Source: CAD feature listing. Evaluate the final solid. Frame: model axes, mm. A direction names the side the tool comes from. Give positions to 0.01 mm unless a question says otherwise; leave off trailing zeros. Order: outer loops, then holes, each group sorted by start corner. A loop starts at its lowest first (then second) coordinate and runs counter-clockwise, first axis right, second up.
from build123d import *

# Parameters (mm, degrees)
PARED_Y_1_4IN_START          = -101.6
CROQUIS1_W                   = 228.6
CROQUIS1_H                   = 50.8
PARED_Y_1_4IN_DEPTH          = 6.35
ROSCA_M3_INFERIOR_START      = 12.7
CROQUIS2_R                   = 1.25
ROSCA_M3_INFERIOR_DEPTH      = 10
ROSCA_M3_SUPERIOR_START      = 53.5
CROQUIS3_R                   = 1.25
ROSCA_M3_SUPERIOR_DEPTH      = 10
BARRENOS_M3_ESQUINAS_START   = -101.6
CROQUIS4_R                   = 1.7
BARRENOS_M3_ESQUINAS_DEPTH   = 6.35
REFRENTADO_M3_ESQUINAS_START = -101.6
CROQUIS5_R                   = 2.9
REFRENTADO_M3_ESQUINAS_DEPTH = 3.2
VENTANA_PUERTOS_RPI5_START   = -101.6
VENTANA_PUERTOS_RPI5_DEPTH   = 6.35
RANURAS_VENTILACION_START    = -101.6
RANURAS_VENTILACION_DEPTH    = 6.35


with BuildPart() as part:
    # Croquis1 → Pared_-Y_1-4in (new body)
    with BuildSketch(Plane(origin=(0, 0, 0), x_dir=(1, 0, 0), z_dir=(0, 1, 0)).offset(PARED_Y_1_4IN_START)):
        with Locations((-25.4, -38.1)):
            Rectangle(CROQUIS1_W, CROQUIS1_H)
    extrude(amount=PARED_Y_1_4IN_DEPTH)

    # Croquis2 → Rosca_M3_inferior (cut)
    with BuildSketch(Plane.XY.offset(ROSCA_M3_INFERIOR_START)):
        with Locations((-125, -98.425)):
            Circle(CROQUIS2_R)
        with Locations((-30, -98.425)):
            Circle(CROQUIS2_R)
        with Locations((70, -98.425)):
            Circle(CROQUIS2_R)
    extrude(amount=ROSCA_M3_INFERIOR_DEPTH, mode=Mode.SUBTRACT)

    # Croquis3 → Rosca_M3_superior (cut)
    with BuildSketch(Plane.XY.offset(ROSCA_M3_SUPERIOR_START)):
        with Locations((-125, -98.425)):
            Circle(CROQUIS3_R)
        with Locations((-30, -98.425)):
            Circle(CROQUIS3_R)
        with Locations((70, -98.425)):
            Circle(CROQUIS3_R)
    extrude(amount=ROSCA_M3_SUPERIOR_DEPTH, mode=Mode.SUBTRACT)

    # Croquis4 → Barrenos_M3_esquinas (cut)
    with BuildSketch(Plane(origin=(0, 0, 0), x_dir=(1, 0, 0), z_dir=(0, 1, 0)).offset(BARRENOS_M3_ESQUINAS_START)):
        with Locations(Location((-136.525, -25, 0), (0, 0, 270))):
            Circle(CROQUIS4_R)
        with Locations(Location((-136.525, -50, 0), (0, 0, 270))):
            Circle(CROQUIS4_R)
        with Locations(Location((85.725, -25, 0), (0, 0, 270))):
            Circle(CROQUIS4_R)
        with Locations(Location((85.725, -50, 0), (0, 0, 270))):
            Circle(CROQUIS4_R)
    extrude(amount=BARRENOS_M3_ESQUINAS_DEPTH, mode=Mode.SUBTRACT)

    # Croquis5 → Refrentado_M3_esquinas (cut)
    with BuildSketch(Plane(origin=(0, 0, 0), x_dir=(1, 0, 0), z_dir=(0, 1, 0)).offset(REFRENTADO_M3_ESQUINAS_START)):
        with Locations(Location((-136.525, -25, 0), (0, 0, 270))):
            Circle(CROQUIS5_R)
        with Locations(Location((-136.525, -50, 0), (0, 0, 270))):
            Circle(CROQUIS5_R)
        with Locations(Location((85.725, -25, 0), (0, 0, 270))):
            Circle(CROQUIS5_R)
        with Locations(Location((85.725, -50, 0), (0, 0, 270))):
            Circle(CROQUIS5_R)
    extrude(amount=REFRENTADO_M3_ESQUINAS_DEPTH, mode=Mode.SUBTRACT)

    # Croquis6 → Ventana_puertos_RPi5 (cut)
    with BuildSketch(Plane(origin=(0, 0, 0), x_dir=(1, 0, 0), z_dir=(0, 1, 0)).offset(VENTANA_PUERTOS_RPI5_START)):
        with BuildLine():
            Line((-108, -47), (-60, -47))
            ThreePointArc((-60, -47), (-57.171572875, -45.828427125), (-56, -43))
            Line((-56, -43), (-56, -24))
            ThreePointArc((-56, -24), (-57.171572875, -21.171572875), (-60, -20))
            Line((-60, -20), (-108, -20))
            ThreePointArc((-108, -20), (-110.828427125, -21.171572875), (-112, -24))
            Line((-112, -24), (-112, -43))
            ThreePointArc((-112, -43), (-110.828427125, -45.828427125), (-108, -47))
        make_face()
    extrude(amount=VENTANA_PUERTOS_RPI5_DEPTH, mode=Mode.SUBTRACT)

    # Croquis7 → Ranuras_ventilacion (cut)
    with BuildSketch(Plane(origin=(0, 0, 0), x_dir=(1, 0, 0), z_dir=(0, 1, 0)).offset(RANURAS_VENTILACION_START)):
        with BuildLine():
            Line((-12, -24.7), (-12, -51.5))
            ThreePointArc((-12, -51.5), (-15, -54.5), (-18, -51.5))
            Line((-18, -51.5), (-18, -24.7))
            ThreePointArc((-18, -24.7), (-15, -21.7), (-12, -24.7))
        make_face()
        with BuildLine():
            Line((3, -24.7), (3, -51.5))
            ThreePointArc((3, -51.5), (0, -54.5), (-3, -51.5))
            Line((-3, -51.5), (-3, -24.7))
            ThreePointArc((-3, -24.7), (0, -21.7), (3, -24.7))
        make_face()
        with BuildLine():
            Line((18, -24.7), (18, -51.5))
            ThreePointArc((18, -51.5), (15, -54.5), (12, -51.5))
            Line((12, -51.5), (12, -24.7))
            ThreePointArc((12, -24.7), (15, -21.7), (18, -24.7))
        make_face()
        with BuildLine():
            Line((33, -24.7), (33, -51.5))
            ThreePointArc((33, -51.5), (30, -54.5), (27, -51.5))
            Line((27, -51.5), (27, -24.7))
            ThreePointArc((27, -24.7), (30, -21.7), (33, -24.7))
        make_face()
        with BuildLine():
            Line((48, -24.7), (48, -51.5))
            ThreePointArc((48, -51.5), (45, -54.5), (42, -51.5))
            Line((42, -51.5), (42, -24.7))
            ThreePointArc((42, -24.7), (45, -21.7), (48, -24.7))
        make_face()
        with BuildLine():
            Line((58, -24.7), (58, -51.5))
            ThreePointArc((58, -51.5), (55, -54.5), (52, -51.5))
            Line((52, -51.5), (52, -24.7))
            ThreePointArc((52, -24.7), (55, -21.7), (58, -24.7))
        make_face()
    extrude(amount=RANURAS_VENTILACION_DEPTH, mode=Mode.SUBTRACT)


solid = part.part
1) Ray query, L1, parallel to Z at x = -62, y = -95.75; L2, parallel to Y at x = 70, z = 18.75 (3 decimals); L3, parallel to Z at x = 12.5, y = -98. Return the intervals inside material, ascending.
Checks:
L1: z = 12.7 to 20, 47 to 63.5
L2: y = -101.6 to -99.675, -97.175 to -95.25
L3: z = 12.7 to 23.04, 53.16 to 63.5
2) Section query A-A on x = 0. Output: boundary loops of the cut face in (y, z), and give its area (3 significant figures).
Checks:
outline: (-101.6, 12.7) - (-95.25, 12.7) - (-95.25, 21.7) - (-101.6, 21.7) - close; (-101.6, 54.5) - (-95.25, 54.5) - (-95.25, 63.5) - (-101.6, 63.5) - close
area: 114 mm2
3) Pull-direction query (Z, two-part tool) for faces 1 (the face through (-84, -98, 47)), 2 (the face through (-27, -98, 12.7)), 3 (the face through (-27, -101.6, 38)); classes: +Z half, -Z half, draft (parallel to the pull), parting line (faces both ways), or undercut.
Checks:
face 1: undercut
face 2: -Z half
face 3: draft
4) Section query B-B on z = 39. State how many separate pieces and enclosed holes the cut face has, and give its area (3 significant figures).
Checks:
separate pieces: 8
enclosed holes: 0
area: 867 mm2
5) First-contact query: pin 1 Ø2 at (x, y) = (-124.5, -98) entering from +Z; pin 2 Ø3 at (x, z) = (86, 49) entering from -Y; pin 3 Ø0.8 at (x, y) = (-29.5, -98) entering from -Z. Flat tips, straight axial feed; report the tip coordinate or a pass-through.
Checks:
pin 1: stops at z = 63.5
pin 2: stops at y = -98.4
pin 3: stops at z = 22.7
6) Reachability of faces 4 (the face through (29.9, -98.5, 21.7)), 5 (the face through (84, -98.4, 51)), 6 (the face through (-139.7, -98, 38)) from +Z, -Z, +X, -X, +Y, -Y: full face, straight path, thin tool, end or side. Return the list, or none.
Checks:
face 4: +Y, -Y
face 5: -Y
face 6: +Z, -Z, -X, +Y, -Y
